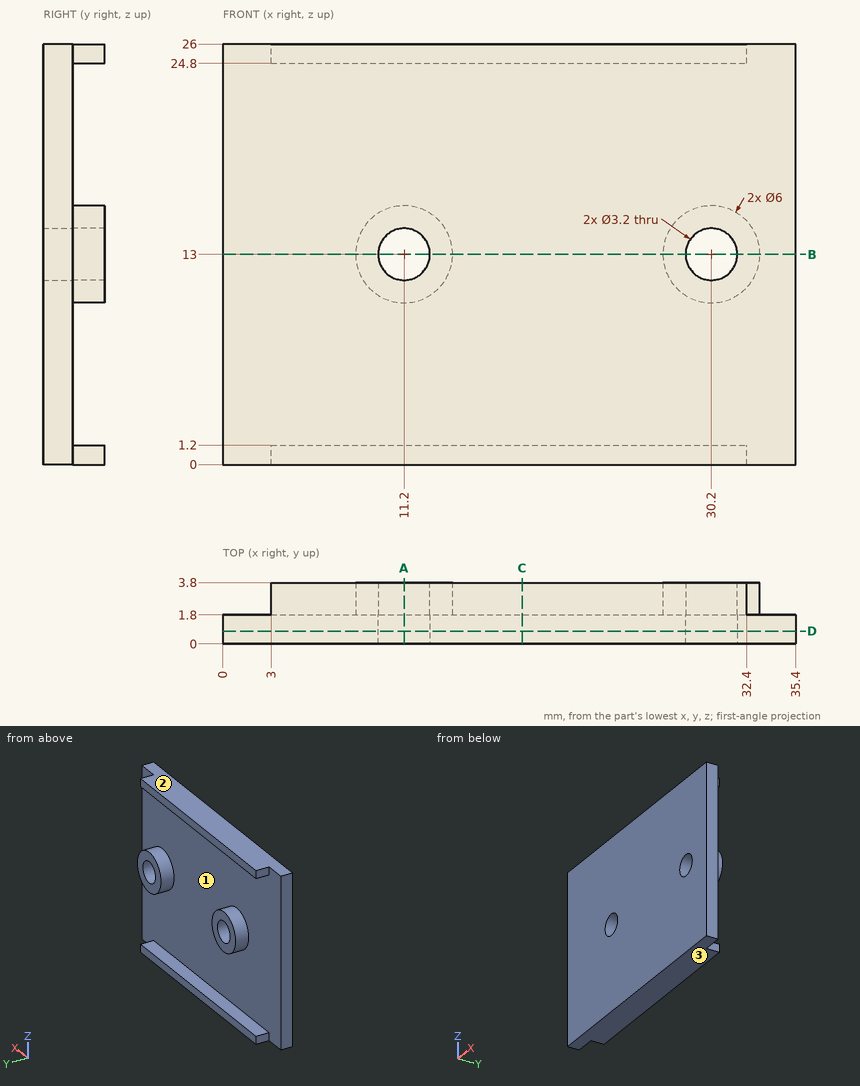
The drawing under review shows one solid part. Ordinate dimensions are in mm from its lowest x, y, z. Coordinates: 2 decimals unless noted, no trailing zeros. Loops run counter-clockwise (first coordinate to the right, second up) from the corner with the lowest first, then second, coordinate; pieces in that order, holes last. Notation, with made-up numbers: (75, 59) -> (125, 59) arc R23 cw to (125, 68) -> close; hole circle Ø10 at (16, 43.25). An arc over 180 degrees is marked (long way). Answer as a JSON object with one key per item and string values.
Q1. Clearance check with flat-ended pins moving along their axes: pin 1 Ø2.5 at (x, z) = (30.2, 13) entering from +Y; pin 2 Ø6 at (x, z) = (26, 18.5) entering from +Y; pin 3 Ø1.3 at (y, z) = (3, 25.5) entering from -X; pin 4 Ø1 at (y, z) = (3, 0.5) entering from +X. State where each tip first meets the part, or that it passes through.
Answer block:
{"pin 1": "passes through", "pin 2": "stops at y = 1.8", "pin 3": "stops at x = 3", "pin 4": "stops at x = 32.4"}
Q2. Take a section at A-A on x = 11.2. Give the boundary of the cut face in (y, z), plus the area to 3 significant figures.
Answer block:
{"outline": "(0, 0) -> (3.8, 0) -> (3.8, 1.2) -> (1.8, 1.2) -> (1.8, 10) -> (3.8, 10) -> (3.8, 11.4) -> (0, 11.4) -> close; (0, 14.6) -> (3.8, 14.6) -> (3.8, 16) -> (1.8, 16) -> (1.8, 24.8) -> (3.8, 24.8) -> (3.8, 26) -> (0, 26) -> close", "area": "51.4 mm^2"}
Q3. Take a section at B-B on z = 13. Give the boundary of the cut face in (x, y), plus the area to 3 significant figures.
Answer block:
{"outline": "(0, 0) -> (9.6, 0) -> (9.6, 3.8) -> (8.2, 3.8) -> (8.2, 1.8) -> (0, 1.8) -> close; (12.8, 0) -> (28.6, 0) -> (28.6, 3.8) -> (27.2, 3.8) -> (27.2, 1.8) -> (14.2, 1.8) -> (14.2, 3.8) -> (12.8, 3.8) -> close; (31.8, 0) -> (35.4, 0) -> (35.4, 1.8) -> (33.2, 1.8) -> (33.2, 3.8) -> (31.8, 3.8) -> close", "area": "63.4 mm^2"}
Q4. To check wall thickness, follow L1, parallel to Z at x = 30.2, y = 2.3; L2, parallel to Z at x = 11.2, y = 0.9; L3, parallel to Z at x = 29, y = 2.9. State the ranges of each line that lie inside material, in increasing order.
Answer block:
{"L1": "z = 0 to 1.2, 10 to 11.4, 14.6 to 16, 24.8 to 26", "L2": "z = 0 to 11.4, 14.6 to 26", "L3": "z = 0 to 1.2, 10.25 to 11.94, 14.06 to 15.75, 24.8 to 26"}
Q5. The part is to be moulded in two halves that separate along Z. For the marked faces 1, 2 and 3, say which applies: +Z half, -Z half, draft (parallel to the pull), parting line (faces both ways), or undercut.
Answer block:
{"face 1": "undercut", "face 2": "+Z half", "face 3": "-Z half"}
Q6. Take a section at C-C on x = 18.5. Give the boundary of the cut face in (y, z).
Answer block:
{"outline": "(0, 0) -> (3.8, 0) -> (3.8, 1.2) -> (1.8, 1.2) -> (1.8, 24.8) -> (3.8, 24.8) -> (3.8, 26) -> (0, 26) -> close"}
Q7. Take a section at D-D on y = 0.8. Give the boundary of the cut face in (x, z), plus the area to 3 significant figures.
Answer block:
{"outline": "(0, 0) -> (35.4, 0) -> (35.4, 26) -> (0, 26) -> close; hole circle Ø3.2 at (11.2, 13); hole circle Ø3.2 at (30.2, 13)", "area": "904 mm^2"}
